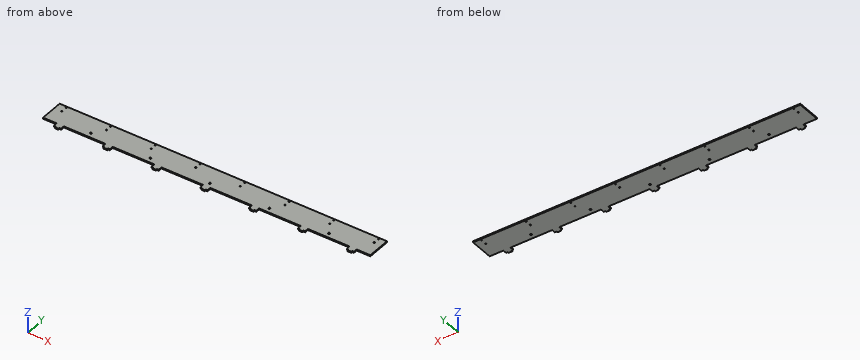
from build123d import *

# Parameters (mm, degrees)
SKETCH_1_W             = 1100
SKETCH_1_H             = 92
EXTRUDE_1_DEPTH        = 2
SKETCH_2_W             = 46
SKETCH_2_H             = 13
SKETCH_2_W_2           = 140
CUT_EXTRUDE_1_DEPTH    = 552.934778756
SKETCH_3_R             = 2
CUT_EXTRUDE_2_DEPTH    = 552.934778756
PATTERN_LINEAR_1_COUNT = 8
PATTERN_LINEAR_1_PITCH = 150
SKETCH_4_R             = 3
CUT_EXTRUDE_3_DEPTH    = 552.934778756
PATTERN_LINEAR_2_COUNT = 5
PATTERN_LINEAR_2_PITCH = 200
SKETCH_5_W             = 12
SKETCH_5_H             = 4
EXTRUDE_2_DEPTH        = 4


with BuildPart() as part:
    # Эскиз1 → Бобышка-Вытянуть1 (new, symmetric)
    with BuildSketch(Plane.XY):
        Rectangle(SKETCH_1_W, SKETCH_1_H)
    extrude(amount=EXTRUDE_1_DEPTH, both=True)

    # Эскиз2 → Вырез-Вытянуть1 (cut, through all)
    with BuildSketch(Plane.XY.offset(2)):
        with Locations((-527, -39.5)):
            Rectangle(SKETCH_2_W, SKETCH_2_H)
        with Locations((527, -39.5)):
            Rectangle(SKETCH_2_W, SKETCH_2_H)
        with Locations((-410, -39.5)):
            Rectangle(SKETCH_2_W_2, SKETCH_2_H)
        with Locations((-246, -39.5)):
            Rectangle(SKETCH_2_W_2, SKETCH_2_H)
        with Locations((-82, -39.5)):
            Rectangle(SKETCH_2_W_2, SKETCH_2_H)
        with Locations((82, -39.5)):
            Rectangle(SKETCH_2_W_2, SKETCH_2_H)
        with Locations((246, -39.5)):
            Rectangle(SKETCH_2_W_2, SKETCH_2_H)
        with Locations((410, -39.5)):
            Rectangle(SKETCH_2_W_2, SKETCH_2_H)
    extrude(amount=-CUT_EXTRUDE_1_DEPTH, mode=Mode.SUBTRACT)

    # Эскиз3 → Вырез-Вытянуть2 (cut, through all)
    with BuildSketch(Plane.XY.offset(2)):
        with Locations((-525, 41)):
            Circle(SKETCH_3_R)
        with Locations((-525, 21)):
            Circle(SKETCH_3_R)
    cut_extrude_2 = extrude(amount=-CUT_EXTRUDE_2_DEPTH, mode=Mode.SUBTRACT)

    # Линейный массив1: Вырез-Вытянуть2 ×8
    with Locations(*[(i * PATTERN_LINEAR_1_PITCH, 0, 0) for i in range(1, PATTERN_LINEAR_1_COUNT)]):
        add(cut_extrude_2, mode=Mode.SUBTRACT)

    # Эскиз4 → Вырез-Вытянуть3 (cut, through all)
    with BuildSketch(Plane(origin=(0, 0, -2), x_dir=(-1, 0, 0), z_dir=(0, 0, -1))):
        with Locations((-399, -16)):
            Circle(SKETCH_4_R)
    cut_extrude_3 = extrude(amount=-CUT_EXTRUDE_3_DEPTH, mode=Mode.SUBTRACT)

    # Линейный массив2: Вырез-Вытянуть3 ×5
    with Locations(*[(-i * PATTERN_LINEAR_2_PITCH, 0, 0) for i in range(1, PATTERN_LINEAR_2_COUNT)]):
        add(cut_extrude_3, mode=Mode.SUBTRACT)

    # Эскиз5 → Бобышка-Вытянуть2 (add)
    with BuildSketch(Plane.XZ.offset(46)):
        with Locations((492, 0)):
            Rectangle(SKETCH_5_W, SKETCH_5_H)
        with Locations((328, 0)):
            Rectangle(SKETCH_5_W, SKETCH_5_H)
        with Locations((164, 0)):
            Rectangle(SKETCH_5_W, SKETCH_5_H)
        Rectangle(SKETCH_5_W, SKETCH_5_H)
        with Locations((-492, 0)):
            Rectangle(SKETCH_5_W, SKETCH_5_H)
        with Locations((-328, 0)):
            Rectangle(SKETCH_5_W, SKETCH_5_H)
        with Locations((-164, 0)):
            Rectangle(SKETCH_5_W, SKETCH_5_H)
    extrude(amount=EXTRUDE_2_DEPTH)


solid = part.part
Part model, mm, in its own coordinate system. Coordinates: 2 decimals unless noted, no trailing zeros. Order: outer loops, then holes, each group sorted by start corner. A loop starts at its lowest first (then second) coordinate and runs counter-clockwise, first axis right, second up.
(1) Slice it at B-B, the plane x = -60. Write the cut outline in (y, z), and give its area (3 significant figures).
Check sheet entries:
outline: (-33, -2) - (46, -2) - (46, 2) - (-33, 2) - close
area: 316 mm2
(2) Probe L1, parallel to Y at x = -75, z = 0; L2, parallel to Y at x = 199, z = -0.65; L3, parallel to Y at x = 305, z = 1.55. List the from-to ranges inside material, lowest first.
Check sheet entries:
L1: y = -33 to 19, 23 to 39, 43 to 46
L2: y = -33 to -19, -13 to 46
L3: y = -33 to 46
(3) Pin check, flat tips, straight feed: pin 1 Ø1.2 at (x, z) = (482.5, -0.5) entering from -Y; pin 2 Ø2 at (y, z) = (-42.5, 0.5) entering from +X; pin 3 Ø1.2 at (y, z) = (-36.5, 0.5) entering from -X. Stop position of each tip, or through.
Check sheet entries:
pin 1: stops at y = -46
pin 2: stops at x = 504
pin 3: stops at x = -504
(4) Slice it at A-A, the plane z = 1.2. State how many separate pieces and enclosed holes the cut face has, and give its area (3 significant figures).
Check sheet entries:
separate pieces: 1
enclosed holes: 21
area: 89,100 mm2
